Autodesk Inventor part; units mm, degrees
ref_plane "YZ Plane" through (0, 0, 0) normal (1, 0, 0) x (0, 1, 0)
ref_plane "XZ Plane" through (0, 0, 0) normal (0, 1, 0) x (-1, 0, 0)
ref_plane "XY Plane" through (0, 0, 0) normal (0, 0, 1) x (1, 0, 0)
sketch "Sketch1" plane through (0, 0, 0) normal (1, 0, 0) x (0, 1, 0)
  line L0 (0, 0) -> (50.8, 0)
  line L1 (50.8, 0) -> (50.8, -38.1)
  line L2 (50.8, -38.1) -> (0, -38.1)
  circle A0 centre (25.4, -19.05) radius 1.651
  line L3 (0, -12.7) -> (2.921, -12.7)
  line L4 (2.921, -12.7) -> (2.921, -25.4)
  line L5 (2.921, -25.4) -> (0, -25.4)
  line L6 (0, -38.1) -> (0, -25.4)
  line L7 (0, -12.7) -> (0, 0)
  dimension "d0" = 50.8
  dimension "d1" = 38.1
  dimension "d2" = 3.302
  dimension "d9" = 12.7
  dimension "d10" = 12.7
  dimension "d11" = 2.921
extrude "Extrusion1" add sketch "Sketch1" along normal blind 2.921
properties part number "wheelsupport"
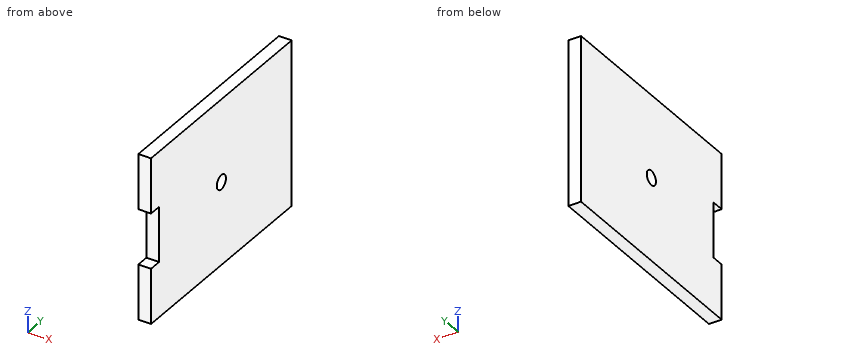
Work out the finished part from the listing and answer in its coordinate system (mm). Give positions to 0.01 mm unless a question says otherwise; leave off trailing zeros. Loops run counter-clockwise (first coordinate to the right, second up) from the corner with the lowest first, then second, coordinate; pieces in that order, holes last. Notation, with made-up numbers: (12.5, 14) -> (70.5, 14) arc R13 ccw to (70.5, 32) -> close; hole circle Ø10 at (85.25, 79). An arc over 180 degrees is marked (long way). Use a Markdown table: item, result. Add a question column.
1) The part is cut by section A-A, the plane y = 25.4. Determine the outline of the cut face in (x, z).
2) The part is cut by section D-D, the plane z = -14.5. Determine the outline of the cut face in (x, y).
3) This flat-tipped pin is pushed along its axis until it touches: P1, Ø1.5, axis at x = 1.5, z = -20, coming from the -Y side. Where does it stop, or does it pass through?
4) Consider line 1 along Z through (x, y) = (1.45, 25.4); line 2 along Y through (x, z) = (0.2, -23). Determine where each line is inside the solid, lowest interval first.
5) The part is cut by section C-C, the plane x = 2.2. Determine the outline of the cut face in (y, z), plus the area to 3 significant figures.
6) The part is cut by section B-B, the plane z = -19.05. Determine the outline of the cut face in (x, y), plus the area to 3 significant figures.
Reported:
| question | item | result |
|---|---|---|
| 1 | outline | (0, -38.1) -> (2.92, -38.1) -> (2.92, -20.7) -> (0, -20.7) -> close; (0, -17.4) -> (2.92, -17.4) -> (2.92, 0) -> (0, 0) -> close |
| 2 | outline | (0, 2.92) -> (2.92, 2.92) -> (2.92, 50.8) -> (0, 50.8) -> close |
| 3 | P1 | stops at y = 2.92 |
| 4 | line 1 | z = -38.1 to -20.7, -17.4 to 0 |
| 4 | line 2 | y = 2.92 to 50.8 |
| 5 | outline | (0, -38.1) -> (50.8, -38.1) -> (50.8, 0) -> (0, 0) -> (0, -12.7) -> (2.92, -12.7) -> (2.92, -25.4) -> (0, -25.4) -> close; hole circle Ø3.3 at (25.4, -19.05) |
| 5 | area | 1,890 mm^2 |
| 6 | outline | (0, 2.92) -> (2.92, 2.92) -> (2.92, 23.75) -> (0, 23.75) -> close; (0, 27.05) -> (2.92, 27.05) -> (2.92, 50.8) -> (0, 50.8) -> close |
| 6 | area | 130 mm^2 |
